from build123d import *
from OCP.BRepFilletAPI import BRepFilletAPI_MakeChamfer

# Parameters (mm, degrees)
SKETCH1_W           = 180
SKETCH1_H           = 180
SKETCH1_R           = 20
SKETCH1_R_2         = 1.6
BOSS_EXTRUDE1_DEPTH = 5
CHAMFER3_SIZE       = 1
CHAMFER3_SIZE2      = 0.577350269
CHAMFER4_SIZE       = 1
CHAMFER4_SIZE2      = 0.577350269


with BuildPart() as part:
    # Sketch1 → Boss-Extrude1 (new body)
    with BuildSketch(Plane(origin=(0, 0, 0), x_dir=(1, 0, 0), z_dir=(0, 1, 0))):
        with Locations((90, 90)):
            Rectangle(SKETCH1_W, SKETCH1_H)
        with Locations(Location((90, 90, 0), (0, 0, 270))):
            Circle(SKETCH1_R, mode=Mode.SUBTRACT)
        with Locations(Location((5, 165, 0), (0, 0, 270))):
            Circle(SKETCH1_R_2, mode=Mode.SUBTRACT)
        with Locations(Location((5, 90, 0), (0, 0, 270))):
            Circle(SKETCH1_R_2, mode=Mode.SUBTRACT)
        with Locations(Location((5, 15, 0), (0, 0, 90))):
            Circle(SKETCH1_R_2, mode=Mode.SUBTRACT)
        with Locations(Location((175, 15, 0), (0, 0, 270))):
            Circle(SKETCH1_R_2, mode=Mode.SUBTRACT)
        with Locations(Location((175, 90, 0), (0, 0, 90))):
            Circle(SKETCH1_R_2, mode=Mode.SUBTRACT)
        with Locations(Location((175, 165, 0), (0, 0, 90))):
            Circle(SKETCH1_R_2, mode=Mode.SUBTRACT)
        with Locations(Location((15, 175, 0), (0, 0, 270))):
            Circle(SKETCH1_R_2, mode=Mode.SUBTRACT)
        with Locations(Location((90, 175, 0), (0, 0, 270))):
            Circle(SKETCH1_R_2, mode=Mode.SUBTRACT)
        with Locations(Location((165, 175, 0), (0, 0, 90))):
            Circle(SKETCH1_R_2, mode=Mode.SUBTRACT)
        with Locations(Location((165, 5, 0), (0, 0, 270))):
            Circle(SKETCH1_R_2, mode=Mode.SUBTRACT)
        with Locations(Location((90, 5, 0), (0, 0, 90))):
            Circle(SKETCH1_R_2, mode=Mode.SUBTRACT)
        with Locations(Location((15, 5, 0), (0, 0, 90))):
            Circle(SKETCH1_R_2, mode=Mode.SUBTRACT)
        with Locations(Location((90, 115, 0), (0, 0, 270))):
            Circle(SKETCH1_R_2, mode=Mode.SUBTRACT)
        with Locations(Location((90, 65, 0), (0, 0, 90))):
            Circle(SKETCH1_R_2, mode=Mode.SUBTRACT)
        with Locations(Location((65, 90, 0), (0, 0, 270))):
            Circle(SKETCH1_R_2, mode=Mode.SUBTRACT)
        with Locations(Location((115, 90, 0), (0, 0, 90))):
            Circle(SKETCH1_R_2, mode=Mode.SUBTRACT)
    extrude(amount=BOSS_EXTRUDE1_DEPTH)

    # Chamfer3
    chamfer3_edges = [part.edges().sort_by_distance(p)[0] for p in [
        (90, 5, -116.6),
        (90, 5, -63.4),
        (65, 5, -91.6),
        (115, 5, -88.4),
    ]]
    chamfer3_side = [part.faces().sort_by_distance(p)[0] for p in [
        (90, 5, -2.545584412),
    ]]
    chamfer(chamfer3_edges, length=CHAMFER3_SIZE, length2=CHAMFER3_SIZE2, reference=chamfer3_side[0])

    # Chamfer4: one chamfer whose edges measure the first distance from different faces: ONE call of the kernel's chamfer builder (chamfer() names one face for all edges)
    chamfer4_edges_1 = [part.edges().sort_by_distance(p)[0] for p in [
        (175, 0, -16.6),
    ]]
    chamfer4_side_1 = [part.faces().sort_by_distance(p)[0] for p in [
        (175, 2.5, -16.6),
    ]]
    chamfer4_edges_2 = [part.edges().sort_by_distance(p)[0] for p in [
        (5, 0, -166.6),
    ]]
    chamfer4_side_2 = [part.faces().sort_by_distance(p)[0] for p in [
        (5, 2.5, -166.6),
    ]]
    chamfer4_edges_3 = [part.edges().sort_by_distance(p)[0] for p in [
        (5, 0, -91.6),
    ]]
    chamfer4_side_3 = [part.faces().sort_by_distance(p)[0] for p in [
        (5, 2.5, -91.6),
    ]]
    chamfer4_edges_4 = [part.edges().sort_by_distance(p)[0] for p in [
        (15, 0, -176.6),
    ]]
    chamfer4_side_4 = [part.faces().sort_by_distance(p)[0] for p in [
        (15, 2.5, -176.6),
    ]]
    chamfer4_edges_5 = [part.edges().sort_by_distance(p)[0] for p in [
        (5, 0, -13.4),
    ]]
    chamfer4_side_5 = [part.faces().sort_by_distance(p)[0] for p in [
        (5, 2.5, -13.4),
    ]]
    chamfer4_edges_6 = [part.edges().sort_by_distance(p)[0] for p in [
        (175, 0, -88.4),
    ]]
    chamfer4_side_6 = [part.faces().sort_by_distance(p)[0] for p in [
        (175, 2.5, -88.4),
    ]]
    chamfer4_edges_7 = [part.edges().sort_by_distance(p)[0] for p in [
        (175, 0, -163.4),
    ]]
    chamfer4_side_7 = [part.faces().sort_by_distance(p)[0] for p in [
        (175, 2.5, -163.4),
    ]]
    chamfer4_edges_8 = [part.edges().sort_by_distance(p)[0] for p in [
        (90, 0, -176.6),
    ]]
    chamfer4_side_8 = [part.faces().sort_by_distance(p)[0] for p in [
        (90, 2.5, -176.6),
    ]]
    chamfer4_edges_9 = [part.edges().sort_by_distance(p)[0] for p in [
        (165, 0, -173.4),
    ]]
    chamfer4_side_9 = [part.faces().sort_by_distance(p)[0] for p in [
        (165, 2.5, -173.4),
    ]]
    chamfer4_edges_10 = [part.edges().sort_by_distance(p)[0] for p in [
        (165, 0, -6.6),
    ]]
    chamfer4_side_10 = [part.faces().sort_by_distance(p)[0] for p in [
        (165, 2.5, -6.6),
    ]]
    chamfer4_edges_11 = [part.edges().sort_by_distance(p)[0] for p in [
        (90, 0, -3.4),
    ]]
    chamfer4_side_11 = [part.faces().sort_by_distance(p)[0] for p in [
        (90, 2.5, -3.4),
    ]]
    chamfer4_edges_12 = [part.edges().sort_by_distance(p)[0] for p in [
        (15, 0, -3.4),
    ]]
    chamfer4_side_12 = [part.faces().sort_by_distance(p)[0] for p in [
        (15, 2.5, -3.4),
    ]]
    chamfer4 = BRepFilletAPI_MakeChamfer(part.part.solid().wrapped)
    for e in chamfer4_edges_1:
        chamfer4.Add(CHAMFER4_SIZE, CHAMFER4_SIZE2, e.wrapped, chamfer4_side_1[0].wrapped)  # the first distance lies on this face
    for e in chamfer4_edges_2:
        chamfer4.Add(CHAMFER4_SIZE, CHAMFER4_SIZE2, e.wrapped, chamfer4_side_2[0].wrapped)  # the first distance lies on this face
    for e in chamfer4_edges_3:
        chamfer4.Add(CHAMFER4_SIZE, CHAMFER4_SIZE2, e.wrapped, chamfer4_side_3[0].wrapped)  # the first distance lies on this face
    for e in chamfer4_edges_4:
        chamfer4.Add(CHAMFER4_SIZE, CHAMFER4_SIZE2, e.wrapped, chamfer4_side_4[0].wrapped)  # the first distance lies on this face
    for e in chamfer4_edges_5:
        chamfer4.Add(CHAMFER4_SIZE, CHAMFER4_SIZE2, e.wrapped, chamfer4_side_5[0].wrapped)  # the first distance lies on this face
    for e in chamfer4_edges_6:
        chamfer4.Add(CHAMFER4_SIZE, CHAMFER4_SIZE2, e.wrapped, chamfer4_side_6[0].wrapped)  # the first distance lies on this face
    for e in chamfer4_edges_7:
        chamfer4.Add(CHAMFER4_SIZE, CHAMFER4_SIZE2, e.wrapped, chamfer4_side_7[0].wrapped)  # the first distance lies on this face
    for e in chamfer4_edges_8:
        chamfer4.Add(CHAMFER4_SIZE, CHAMFER4_SIZE2, e.wrapped, chamfer4_side_8[0].wrapped)  # the first distance lies on this face
    for e in chamfer4_edges_9:
        chamfer4.Add(CHAMFER4_SIZE, CHAMFER4_SIZE2, e.wrapped, chamfer4_side_9[0].wrapped)  # the first distance lies on this face
    for e in chamfer4_edges_10:
        chamfer4.Add(CHAMFER4_SIZE, CHAMFER4_SIZE2, e.wrapped, chamfer4_side_10[0].wrapped)  # the first distance lies on this face
    for e in chamfer4_edges_11:
        chamfer4.Add(CHAMFER4_SIZE, CHAMFER4_SIZE2, e.wrapped, chamfer4_side_11[0].wrapped)  # the first distance lies on this face
    for e in chamfer4_edges_12:
        chamfer4.Add(CHAMFER4_SIZE, CHAMFER4_SIZE2, e.wrapped, chamfer4_side_12[0].wrapped)  # the first distance lies on this face
    add(Compound.cast(chamfer4.Shape()), mode=Mode.REPLACE)


solid = part.part
Input: part model. Units: mm. Frame: model coordinates. Coordinates: 2 decimals unless noted, no trailing zeros. Loops run counter-clockwise (first coordinate to the right, second up) from the corner with the lowest first, then second, coordinate; pieces in that order, holes last.
Q1. Material intervals for line 1 (X direction, y = 2.25, z = -175); line 2 (Z direction, x = 175, y = 3.5); line 3 (X direction, y = 1.7, z = -115), sorted ascending.
Q2. Cut plane A-A (y = 2.3). Give the number of separate pieces and of enclosed holes in the cut face, then the cut area to 3 significant figures.
Q3. Draft query along X for faces 1 (the face through (0, 2, -89)), 2 (the face through (89, 2, 0)), 3 (the face through (180, 2, -89)). Return one class per face: +X half, -X half, draft (parallel to the pull), parting line (faces both ways), or undercut.
Q4. Contact query for flat-ended pins moving along their axis: pin 1 (3 mm diameter, centred on x = 5, z = -165, fed in from -Y); pin 2 (4 mm diameter, centred on x = 90, z = -65, fed in from +Y); pin 3 (4 mm diameter, centred on x = 165, z = -5, fed in from -Y); pin 4 (3.5 mm diameter, centred on x = 165, z = -175, fed in from -Y). Output: stop coordinate, or through.
Q5. Cut plane B-B (z = -104.5). Output: boundary loops of the cut face in (x, y), then the cut area to 3 significant figures.
Working result:
1. line 1: x = 0 to 13.4, 16.6 to 88.4, 91.6 to 163.4, 166.6 to 180
1. line 2: z = -180 to -166.6, -163.4 to -91.6, -88.4 to -16.6, -13.4 to 0
1. line 3: x = 0 to 88.4, 91.6 to 180
2. separate pieces: 1
2. enclosed holes: 17
2. area: 31,000 mm2
3. face 1: -X half
3. face 2: draft
3. face 3: +X half
4. pin 1: passes through
4. pin 2: stops at y = 4.65
4. pin 3: stops at y = 0.31
4. pin 4: stops at y = 0.74
5. outline: (0, 0) - (76.23, 0) - (76.23, 5) - (0, 5) - close; (103.77, 0) - (180, 0) - (180, 5) - (103.77, 5) - close
5. area: 762 mm2
